Autodesk Inventor part; units mm, degrees
ref_plane "YZ Plane" through (0, 0, 0) normal (1, 0, 0) x (0, 1, 0)
ref_plane "XZ Plane" through (0, 0, 0) normal (0, 1, 0) x (-1, 0, 0)
ref_plane "XY Plane" through (0, 0, 0) normal (0, 0, 1) x (1, 0, 0)
sketch "Sketch1" plane through (0, 0, 0) normal (0, 0, 1) x (1, 0, 0)
  line L0 (0, 0) -> (-1.6865, 12)
  line L1 (-1.6865, 12) -> (0, 12)
  line L2 (0, 12) -> (0, 0)
  dimension "d0" = 8
  dimension "d1" = 12
extrude "Extrusion1" add sketch "Sketch1" along normal blind 175
sketch "Sketch2" plane through (0, 0, 175) normal (0, 0, 1) x (1, 0, 0)
  line L0 (0, 0) -> (0, 12)
  line L1 (0, 12) -> (-1.6865, 12)
  line L2 (0, 12) -> (2, 12)
  line L3 (2, 12) -> (2.3, 12.3)
  line L4 (2.3, 12.3) -> (4, 12.3)
  line L5 (4, 12.3) -> (4, 10.8)
  line L6 (4, 10.8) -> (0, 10.8)
  line L7 (0, 7.2) -> (4, 7.2)
  line L8 (4, 7.2) -> (4, 5.7)
  line L9 (4, 5.7) -> (2.3, 5.7)
  line L10 (2.3, 5.7) -> (2, 6)
  line L11 (2, 6) -> (0, 6)
  dimension "d4" = 2
  dimension "d5" = 4
  dimension "d6" = 135
  dimension "d9" = 135
  dimension "d17" = 6
  dimension "d18" = 6.6
  dimension "d19" = 1.2
extrude "Extrusion2" add sketch "Sketch2" against normal blind 20
pattern_linear "Rectangular Pattern1" count 3 spacing 77.5 along (0, 0, -1) of "Extrusion2"
properties part number "LedStripHolder"
Check sheet for the modelled part. Datum: model origin and axes. Units: mm. A direction names the side the tool comes from. Round coordinates to 2 decimals unless told otherwise and drop trailing zeros. Loops run counter-clockwise (first coordinate to the right, second up) from the corner with the lowest first, then second, coordinate; pieces in that order, holes last. Notation, with made-up numbers: (-11, 87) - (46, 87) arc R37 cw to (46, 125) - close; hole circle Ø8 at (64, 82). An arc over 180 degrees is marked (long way). Answer as CSV lines item,"result". Start each with the question number.
Item 1: Section check B-B (z = 94). Record the boundary of the cut face in (x, y), and give its area (3 significant figures).
Item 2: Section check D-D (z = 120). Record the boundary of the cut face in (x, y).
Item 3: Depth check by flat-ended pin: P1, Ø5, axis at y = 1.5, z = 45, coming from the +X side; P2, Ø3, axis at y = 3, z = 96, coming from the -X side; P3, Ø0.8, axis at x = 3, z = 166, coming from the -Y side; P4, Ø1.5, axis at x = 2, z = 121.5, coming from the -Y side (3 decimals). Enter the tip coordinate at first touch or a pass-through.
Item 4: Scan lines: line 1 (Z direction, x = 2.3, y = 6.5); line 2 (Y direction, x = 2, z = 84); line 3 (X direction, y = 9, z = 72). Record each from-to range of solid material in increasing order. Write a range as [from, to].
Item 5: Set-up check for faces 5 (the flat face through (-0.83, 5.92, 86.28)), 6 (the flat face through (2, 10.8, 10)): record each of +Z, -Z, +X, -X, +Y, -Y from which the full face is reachable in a straight line by a thin tool's end or side.
Item 6: Release check for a two-part mould opening along Z. For faces 1 (the flat face through (1, 7, 0)), 2 (the flat face through (0, 5, 86)), 3 (the flat face through (0, 12, 86)), 4 (the flat face through (1, 7, 175)) record: +Z half, -Z half, draft (parallel to the pull), parting line (faces both ways), or undercut.
Item 7: Section check A-A (x = 0.9). Record the boundary of the cut face in (y, z), and give its area (3 significant figures).
Item 8: Section check C-C (y = 4.25). Record the boundary of the cut face in (x, z), and give its area (3 significant figures).
Report:
1,outline,"(-1.69, 12) - (0, 0) - (0, 6) - (2, 6) - (2.3, 5.7) - (4, 5.7) - (4, 7.2) - (0, 7.2) - (0, 10.8) - (4, 10.8) - (4, 12.3) - (2.3, 12.3) - (2, 12) - close"
1,area,"20.8 mm2"
2,outline,"(-1.69, 12) - (0, 0) - (0, 12) - close"
3,P1,"stops at x = 0"
3,P2,"stops at x = -0.63"
3,P3,"stops at y = 5.7"
3,P4,"passes through"
4,line 1,"z = [0, 20], [77.5, 97.5], [155, 175]"
4,line 2,"y = [6, 7.2], [10.8, 12]"
4,line 3,"x = [-1.26, 0]"
5,face 5,"+Z, -Z, -X, -Y"
5,face 6,"+Z, -Z, +X"
6,face 1,"-Z half"
6,face 2,"undercut"
6,face 3,"draft"
6,face 4,"+Z half"
7,outline,"(6, 0) - (7.2, 0) - (7.2, 20) - (6, 20) - close; (6, 77.5) - (7.2, 77.5) - (7.2, 97.5) - (6, 97.5) - close; (6, 155) - (7.2, 155) - (7.2, 175) - (6, 175) - close; (10.8, 0) - (12, 0) - (12, 20) - (10.8, 20) - close; (10.8, 77.5) - (12, 77.5) - (12, 97.5) - (10.8, 97.5) - close; (10.8, 155) - (12, 155) - (12, 175) - (10.8, 175) - close"
7,area,"144 mm2"
8,outline,"(-0.6, 0) - (0, 0) - (0, 175) - (-0.6, 175) - close"
8,area,"105 mm2"
